from build123d import *

# Parameters (mm, degrees)
F0_W     = 3
F0_H     = 3
F0_W_2   = 22
F0_H_2   = 24
F0_W_3   = 17
F1_DEPTH = 12.5
F2_R     = 10
F3_R     = 5


with BuildPart() as f1:
    # F0 (on Front) → F1 (new body, symmetric)
    with BuildSketch(Plane.XZ):
        with Locations((1.5, 1.5)):
            Rectangle(F0_W, F0_H)
        with Locations((14, 1.5)):
            Rectangle(F0_W_2, F0_H)
        with Locations((1.5, 15)):
            Rectangle(F0_W, F0_H_2)
        with Locations((1.5, 28.5)):
            Rectangle(F0_W, F0_H)
        with Locations((11.5, 28.5)):
            Rectangle(F0_W_3, F0_H)
    extrude(amount=F1_DEPTH, both=True)

    # F2
    f2_edges = [f1.edges().sort_by_distance(p)[0] for p in [
        (20, -12.5, 28.5),
        (20, 12.5, 28.5),
    ]]
    fillet(f2_edges, radius=F2_R)

    # F3
    f3_edges = [f1.edges().sort_by_distance(p)[0] for p in [
        (25, -12.5, 1.5),
        (25, 12.5, 1.5),
    ]]
    fillet(f3_edges, radius=F3_R)


solid = f1.part
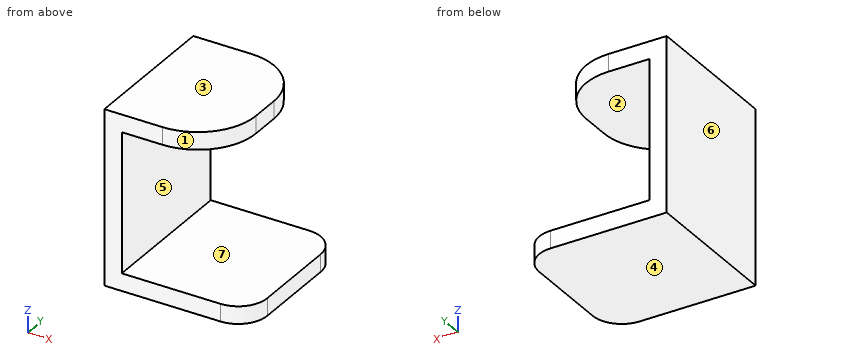
Design review of the part built by this model. Coordinates are the model's own, in mm. Face numbers are marked on the shaded views. A direction names the side the tool comes from. Coordinates: 2 decimals unless noted, no trailing zeros. Order: outer loops, then holes, each group sorted by start corner. A loop starts at its lowest first (then second) coordinate and runs counter-clockwise, first axis right, second up. Notation, with made-up numbers: (51.5, 71.5) -> (99.5, 71.5) arc R24 cw to (99.5, 97.5) -> close; hole circle Ø6 at (81.25, 25). An arc over 180 degrees is marked (long way). Use one line per item in the form item = value. Start each with the question number.
(1) Add section D-D on x = 10.75. State the section outline as (y, z) points, plus the area to 3 significant figures.
(2) Insertion check: pin 1 (12 mm diameter, centred on y = -6, z = 16.5, fed in from +X); pin 2 (12 mm diameter, centred on x = 19.5, z = 15.5, fed in from -Y); pin 3 (0.9 mm diameter, centred on y = 1, z = 29, fed in from +X). Each pin has a flat end and moves straight along its axis. Give the tip position at first contact, or say it passes through.
(3) Add section C-C on z = 2.5. State the section outline as (x, y) points, plus the area to 3 significant figures.
(4) For the marked faces 1, 2 and 3, list the 3-axis set-ups (+Z, -Z, +X, -X, +Y, -Y) from which the entire face can be reached by the end or side of a thin tool; tool diameter is ignored.
(5) For probe 1 along Z at (x, y) = (10.5, -2.5); probe 2 along X at (y, z) = (-5, 22.25), list the stretches that pass through material, from the lowest coordinate up.
(6) The part is to be moulded in two halves that separate along Z. For the marked faces 4, 5, 6 and 7, say which applies: +Z half, -Z half, draft (parallel to the pull), parting line (faces both ways), or undercut.
(7) Add section A-A on x = 5.25. State the section outline as (y, z) points.
(8) Add section B-B on y = -0.5. State the section outline as (x, z) points, plus the area to 3 significant figures.
Answer block:
q1.outline = (-12.5, 0) -> (12.5, 0) -> (12.5, 3) -> (-12.5, 3) -> close; (-12.47, 27) -> (12.47, 27) -> (12.47, 30) -> (-12.47, 30) -> close
q1.area = 150 mm²
q2.pin_1 = 3
q2.pin_2 = through
q2.pin_3 = 20
q3.outline = (0, -12.5) -> (20, -12.5) arc R5 ccw to (25, -7.5) -> (25, 7.5) arc R5 ccw to (20, 12.5) -> (0, 12.5) -> close
q3.area = 614 mm²
q4.face_1 = +Z, +X, -Y
q4.face_2 = +X, +Y, -Y
q4.face_3 = +Z, +X, -X, +Y, -Y
q5.probe_1 = 0 to 3, 27 to 30
q5.probe_2 = 0 to 3
q6.face_4 = -Z half
q6.face_5 = undercut
q6.face_6 = draft
q6.face_7 = undercut
q7.outline = (-12.5, 0) -> (12.5, 0) -> (12.5, 3) -> (-12.5, 3) -> close; (-12.5, 27) -> (12.5, 27) -> (12.5, 30) -> (-12.5, 30) -> close
q8.outline = (0, 0) -> (25, 0) -> (25, 3) -> (3, 3) -> (3, 27) -> (20, 27) -> (20, 30) -> (0, 30) -> close
q8.area = 207 mm²
